from build123d import *

# Parameters (mm, degrees)
F0_W      = 38.1
F0_H      = 38.1
F1_DEPTH  = 38.1
F6_DEPTH  = 38.1
F8_DEPTH  = 38.1
F9_W      = 25.4
F9_H      = 7.62
F10_DEPTH = 38.1


with BuildPart() as f1:
    # F0 (on Front) → F1 (new body)
    with BuildSketch(Plane.XZ):
        with Locations((19.05, 19.05)):
            Rectangle(F0_W, F0_H)
    extrude(amount=F1_DEPTH)

    # F5 (on offset) → F6 (cut)
    with BuildSketch(Plane.YZ.offset(38.1)):
        Polygon((-38.1, 0), (-31.75, 0), (-38.1, 38.1), align=None)
        Polygon((-12.7, 18.439805), (-6.35, 38.1), (-31.75, 38.1), (-26.67, 18.439805), (-21.59, 33.184951), (-16.51, 33.184951), align=None)
        Polygon((-25.4, 0), (-12.7, 0), (-19.05, 15.875), align=None)
        Polygon((-6.35, 0), (0, 0), (0, 38.1), align=None)
    extrude(amount=-F6_DEPTH, mode=Mode.SUBTRACT)

    # F7 (on offset) → F8 (cut)
    with BuildSketch(Plane.XZ.offset(38.1)):
        Polygon((0, 38.1), (0, 0), (6.35, 38.1), align=None)
        Polygon((11.43, 22.225), (6.35, 0), (31.75, 0), (26.67, 22.225), (21.59, 9.525), (16.51, 9.525), align=None)
        Polygon((25.4, 38.1), (12.7, 38.1), (19.05, 22.225), align=None)
        Polygon((31.75, 38.1), (38.1, 0), (38.1, 38.1), align=None)
    extrude(amount=-F8_DEPTH, mode=Mode.SUBTRACT)

    # F9 (on offset) → F10 (cut)
    with BuildSketch(Plane.XY.offset(38.1)):
        with Locations((25.4, -11.43)):
            Rectangle(F9_W, F9_H)
        with Locations((12.7, -26.67)):
            Rectangle(F9_W, F9_H)
    extrude(amount=-F10_DEPTH, mode=Mode.SUBTRACT)


solid = f1.part
The listing builds one solid part. Answer for the finished solid, in the listing's coordinates (mm). A direction names the side the tool comes from. Give positions to 0.01 mm unless a question says otherwise; leave off trailing zeros. Write each loop counter-clockwise with the first axis right and the second up, starting at its lowest first coordinate (ties: lowest second). Pieces come first, ordered by that corner, then holes.
1) Find the intervals of material crossed by L1, parallel to X at y = -7, z = 18.5; L2, parallel to Y at x = 28.5, z = 29; L3, parallel to Y at x = 10.5, z = 27, in increasing order.
2) A tool of negligible diameter and unlimited length cuts with its end or side. For faces 4 (the face through (32.6, -17.1, 11)), 5 (the face through (13, -30.48, 21)), 6 (the face through (15.83, -4.71, 30.27)), from which of +Z, -Z, +X, -X, +Y, -Y can it reach the whole face along a straight path? Write none if from no direction.
3) For a pull along X with two mould halves and no side action, classify faces 1 (the face through (33.2, -22.2, 8)), 2 (the face through (13.44, -19.04, 17.2)), 3 (the face through (12.7, -15, 22)) as pulls with the +X half, pulls with the -X half, needs draft (parallel to the pull), parting line crosses it, or undercut.
4) Section B-B (z = 7) is taken. Write down the section's boundary in (x, y), and give its area (3 significant figures).
5) Given P1, Ø12, axis at y = -27, z = 13, coming from the +X side; P2, Ø6, axis at y = -5, z = 21, coming from the +X side; P3, Ø1.9, axis at y = -14, z = 21.5, coming from the +X side, each flat-ended and moving along its own axis, determine where each tip first touches the part or whether it passes through.
6) Section D-D (y = -18.5) is taken. Write down the section's boundary in (x, z) (3 decimals).
7) Section A-A (x = 18.5) is taken. Count the separate pieces of the cut face and the enclosed holes in it, and give its area (3 significant figures).
Response:
1. L1: x = 3.08 to 10.58, 12.92 to 25.18, 27.52 to 35.02
1. L2: y = -36.58 to -29.4, -23.03 to -15.43, -7.62 to -1.52
1. L3: y = -36.25 to -30.48, -22.86 to -14.91, -9.94 to -1.85
2. face 4: -Z, +X, -X
2. face 5: +Z, -Z, -X
2. face 6: +Z, +Y, -Y
3. face 1: needs draft
3. face 2: undercut
3. face 3: pulls with the +X half
4. outline: (1.17, -32.92) - (7.95, -32.92) - (7.95, -30.48) - (1.17, -30.48) - close; (1.17, -22.86) - (7.95, -22.86) - (7.95, -22.6) - (1.17, -22.6) - close; (1.17, -15.5) - (7.95, -15.5) - (7.95, -5.18) - (1.17, -5.18) - close; (30.15, -32.92) - (36.93, -32.92) - (36.93, -22.6) - (30.15, -22.6) - close; (30.15, -15.5) - (36.93, -15.5) - (36.93, -15.24) - (30.15, -15.24) - close; (30.15, -7.62) - (36.93, -7.62) - (36.93, -5.18) - (30.15, -5.18) - close
4. area: 177 mm2
5. P1: stops at x = 36.93
5. P2: stops at x = 35.1
5. P3: stops at x = 12.7
6. outline: (2.417, 14.5) - (9.664, 14.5) - (11.43, 22.225) - (14.52, 14.5) - (23.58, 14.5) - (26.67, 22.225) - (28.436, 14.5) - (35.683, 14.5) - (32.569, 33.185) - (23.434, 33.185) - (19.05, 22.225) - (14.666, 33.185) - (5.531, 33.185) - close
7. separate pieces: 3
7. enclosed holes: 0
7. area: 205 mm2
